from build123d import *

# Parameters (mm, degrees)
EXTRUDE018_DEPTH                          = 25.4
EXTRUDE018_ONTO_SKETCH024_PLACEMENT_ANGLE = 8
SKETCH018_AS_DRAWN_R                      = 1.2
EXTRUDE009_DEPTH                          = 7.8
EXTRUDE009_ONTO_SKETCH018_PLACEMENT_ANGLE = 8
EXTRUDE010_DEPTH                          = 1.4
EXTRUDE010_ONTO_SKETCH019_PLACEMENT_ANGLE = 8


with BuildPart() as reset_switch_hole:
    # Sketch024 as drawn → Extrude018 (new, symmetric)
    with BuildSketch(Plane.XY):
        Polygon((-152.83455, 73.27651), (-140.412076, 70.636031), (-143.052554, 58.213557), (-155.475029, 60.854035), align=None)
    extrude(amount=EXTRUDE018_DEPTH, both=True)


with BuildPart() as reset_switch_hole_1:
    # Extrude018 onto Sketch024 placement: moved
    add(reset_switch_hole.part.moved(Location((-7.384231, 0, 52.541536))).rotate(Axis((-7.384231, 0, 52.541536), (0, -1, 0)), EXTRUDE018_ONTO_SKETCH024_PLACEMENT_ANGLE))


with BuildPart() as screw_hole_cuts:
    # Sketch018 as drawn → Extrude009 (new)
    with BuildSketch(Plane.XY):
        with Locations((-31.998318, 84.649891)):
            Circle(SKETCH018_AS_DRAWN_R)
        with Locations((-31.998318, -89.695043)):
            Circle(SKETCH018_AS_DRAWN_R)
        with Locations((156.654735, -49.595599)):
            Circle(SKETCH018_AS_DRAWN_R)
        with Locations((156.654735, 84.649891)):
            Circle(SKETCH018_AS_DRAWN_R)
    extrude(amount=EXTRUDE009_DEPTH)


with BuildPart() as screw_hole_cuts_1:
    # Extrude009 onto Sketch018 placement: moved
    add(screw_hole_cuts.part.moved(Location((39.98734, 0, 30.691416))).rotate(Axis((39.98734, 0, 30.691416), (0, 1, 0)), EXTRUDE009_ONTO_SKETCH018_PLACEMENT_ANGLE))


with BuildPart() as right_plate_solid_w_screw_holes:
    # Sketch019 as drawn → Extrude010 (new)
    with BuildSketch(Plane.XY):
        with BuildLine():
            Line((-37.205318, 86.681891), (-37.205318, -92.017095))
            ThreePointArc((-37.205318, -92.017095), (-36.028411, -94.484534), (-33.370199, -95.122714))
            Line((-33.370199, -95.122714), (159.34685, -54.159441))
            ThreePointArc((159.34685, -54.159441), (161.154172, -53.051915), (161.861735, -51.053821))
            Line((161.861735, -51.053821), (161.861735, 86.681892))
            ThreePointArc((161.861735, 86.681892), (160.931799, 88.926956), (158.686734, 89.856891))
            Line((158.686734, 89.856891), (-34.030318, 89.856891))
            ThreePointArc((-34.030318, 89.856891), (-36.275382, 88.926955), (-37.205318, 86.681891))
        make_face()
    extrude(amount=EXTRUDE010_DEPTH)


with BuildPart() as right_plate_solid_w_screw_holes_1:
    # Extrude010 onto Sketch019 placement: moved
    add(right_plate_solid_w_screw_holes.part.moved(Location((39.98734, 0, 30.691416))).rotate(Axis((39.98734, 0, 30.691416), (0, 1, 0)), EXTRUDE010_ONTO_SKETCH019_PLACEMENT_ANGLE))

    # Cut002: cut Screw Hole Cuts
    add(screw_hole_cuts_1.part, mode=Mode.SUBTRACT)


with BuildPart() as cut011:
    # Part__Mirroring003: instance of Right Plate Solid w/ Screw Holes
    add(right_plate_solid_w_screw_holes_1.part.mirror(Plane(origin=(0, 0, 0), x_dir=(0, -1, 0), z_dir=(1, 0, 0))))

    # Cut011: cut Reset Switch Hole
    add(reset_switch_hole_1.part, mode=Mode.SUBTRACT)


solid = cut011.part
Source: CAD feature listing. Evaluate the final solid. Frame: model axes, mm. Coordinates: 2 decimals unless noted, no trailing zeros. Order: outer loops, then holes, each group sorted by start corner. A loop starts at its lowest first (then second) coordinate and runs counter-clockwise, first axis right, second up. Notation, with made-up numbers: M -23,9.25 L 13,9.25 A13 ccw 13,29.25 Z; hole C 27.25,42.25 d2. An arc over 180 degrees is marked long. Write each question's results on one line, items separated by ' | '. Start each with the question number.
1. Section C-C, the plane y = 27.5. Return the cut outline in (x, z), then the cut area to 3 significant figures.
2. Section A-A, the plane y = 64. Return the cut outline in (x, z).
3. Pin query (flat end, axial travel): pin 1 (6 mm diameter, centred on x = -131, z = 19, fed in from -Y); pin 2 (2 mm diameter, centred on x = -155, y = 34.5, fed in from +Z); pin 3 (6 mm diameter, centred on x = -99, z = 21.5, fed in from +Y); pin 4 (5 mm diameter, centred on x = -32, y = -36.5, fed in from +Z). Return the tip coordinate at first contact, or that it passes through.
4. Section B-B, the plane z = 20. Return the cut outline in (x, y).
5. Material intervals for L1, parallel to Z at x = -190.5, y = -31.5; L2, parallel to Z at x = -144, y = 54.5, sorted ascending.
Solution:
1) outline: M -200.47,9.55 L -200.27,8.16 L -3.14,35.87 L -3.34,37.26 Z | area: 279 mm²
2) outline: M -200.47,9.55 L -200.27,8.16 L -158.3,14.06 L -158.5,15.45 Z; M -145.64,17.26 L -145.45,15.87 L -3.14,35.87 L -3.34,37.26 Z
3) pin 1: y = -69.16 | pin 2: z = 16.08 | pin 3: y = 89.86 | pin 4: z = 33.58
4) outline: M -126.12,-69.58 L -116.06,-71.7 L -116.06,89.86 L -126.12,89.86 Z
5) L1: 9.54 to 10.95 | L2: 16.07 to 17.49
